Could you check a few things on this model? Use its own coordinates, in mm. A direction names the side the tool comes from. Round coordinates to 2 decimals unless told otherwise and drop trailing zeros. Loops run counter-clockwise (first coordinate to the right, second up) from the corner with the lowest first, then second, coordinate; pieces in that order, holes last. Notation, with made-up numbers: (88.5, 17) -> (143.5, 17) arc R13 ccw to (143.5, 30) -> close; hole circle Ø8 at (76.5, 40.25). An arc over 180 degrees is marked (long way). Write each question's results on one line, items separated by ' | '.
from build123d import *

# Parameters (mm, degrees)
F0_W     = 61.1153859645
F0_H     = 51.6923125833
F1_DEPTH = 20
F2_W     = 57.1153859645
F2_H     = 47.6923125833
F3_DEPTH = 19
F4_R     = 2.5
F4_R_2   = 1.5
F5_DEPTH = 10
F6_DEPTH = 1


# Not quite as in the source:
# - a feature of the source that left no trace in its solid (it failed there, or was rolled back) is left out


with BuildPart() as f1:
    # F0 (on Top) → F1 (new body)
    with BuildSketch(Plane.XY):
        with Locations((-0.1346161589, -0.9423075244)):
            Rectangle(F0_W, F0_H)
    extrude(amount=F1_DEPTH)

    # F2 (on face) → F3 (cut)
    with BuildSketch(Plane(origin=(0, 0, 0), x_dir=(1, 0, 0), z_dir=(0, 0, -1))):
        with Locations((-0.1346161589, 0.9423075244)):
            Rectangle(F2_W, F2_H)
    extrude(amount=-F3_DEPTH, mode=Mode.SUBTRACT)

    # F4 (on face) → F5 (join)
    with BuildSketch(Plane(origin=(0, 0, 19), x_dir=(1, 0, 0), z_dir=(0, 0, -1))):
        with Locations((-10.9730726108, -8.6767822504)):
            Circle(F4_R)
        with Locations((-10.9730726108, -8.6767822504)):
            Circle(F4_R_2, mode=Mode.SUBTRACT)
        with Locations((5.6683224998, 9.3844144205)):
            Circle(F4_R)
        with Locations((5.6683224998, 9.3844144205)):
            Circle(F4_R_2, mode=Mode.SUBTRACT)
    extrude(amount=F5_DEPTH)

    # F6 (cut): faces of the model
    f6_faces = [f1.faces().sort_by_distance(p)[0] for p in [
        (-10.9730726108, 8.6767822504, 19),
        (5.6683224998, -9.3844144205, 19),
    ]]
    extrude(f6_faces, amount=-F6_DEPTH, mode=Mode.SUBTRACT)


solid = f1.part
1) If we mould it in two halves opening along X, with no side actions, what happens to faces 3 (the flat face through (-1, -1, 20)), 4 (the flat face through (-30.692, -1, 10)), 5 (the cylindrical face through (-11.3, 6.2, 14.1))? For each: released by +X, released by -X, zero draft, split by the parting line, or undercut.
Model answer:
face 3: zero draft | face 4: released by -X | face 5: undercut
2) I'm going to push flat-ended pins straight in: pin 1 (5.5 mm diameter, centred on x = 6, y = -10, fed in from -Z); pin 2 (4 mm diameter, centred on x = -5, y = 9.5, fed in from -Z). Where does each tip first touch, or does it pass through?
Model answer:
pin 1: stops at z = 9 | pin 2: stops at z = 19
3) For faces 1 (the cylindrical face through (8.05, -10.14, 14.07)), 2 (the flat face through (30.423, -1, 10)), which set-ups out of +Z, -Z, +X, -X, +Y, -Y let a thin tool reach every point of the face, with its end or its side?
Model answer:
face 1: -Z | face 2: +Z, -Z, +X, +Y, -Y
4) I need wall thicknesses on line 1 (Y direction, x = 25, z = 2.25); line 2 (X direction, y = -14.5, z = 11.25); line 3 (Z direction, x = 11, y = -21). Which ranges of each line are inside material? Lowest first, please.
Model answer:
line 1: y = -26.79 to -24.79, 22.9 to 24.9 | line 2: x = -30.69 to -28.69, 28.42 to 30.42 | line 3: z = 19 to 20
5) I want a section at A-A, the plane z = 12. Write out the boundary of the cut face in (x, y), plus the area to 3 significant figures.
Model answer:
outline: (-30.69, -26.79) -> (30.42, -26.79) -> (30.42, 24.9) -> (-30.69, 24.9) -> close; circle Ø5 at (-10.97, 8.68); circle Ø5 at (5.67, -9.38); hole (-28.69, -24.79) -> (28.42, -24.79) -> (28.42, 22.9) -> (-28.69, 22.9) -> close; hole circle Ø3 at (-10.97, 8.68); hole circle Ø3 at (5.67, -9.38) | area: 460 mm2
6) I want a section at B-B, the plane z = 7.25. Write out the boundary of the cut face in (x, y).
Model answer:
outline: (-30.69, -26.79) -> (30.42, -26.79) -> (30.42, 24.9) -> (-30.69, 24.9) -> close; hole (-28.69, -24.79) -> (28.42, -24.79) -> (28.42, 22.9) -> (-28.69, 22.9) -> close
7) I want a section at D-D, the plane x = 21. Write out the boundary of the cut face in (y, z), plus the area to 3 significant figures.
Model answer:
outline: (-26.79, 0) -> (-24.79, 0) -> (-24.79, 19) -> (22.9, 19) -> (22.9, 0) -> (24.9, 0) -> (24.9, 20) -> (-26.79, 20) -> close | area: 128 mm2
8) I want a section at C-C, the plane y = -5. Write out the boundary of the cut face in (x, z).
Model answer:
outline: (-30.69, 0) -> (-28.69, 0) -> (-28.69, 19) -> (28.42, 19) -> (28.42, 0) -> (30.42, 0) -> (30.42, 20) -> (-30.69, 20) -> close
